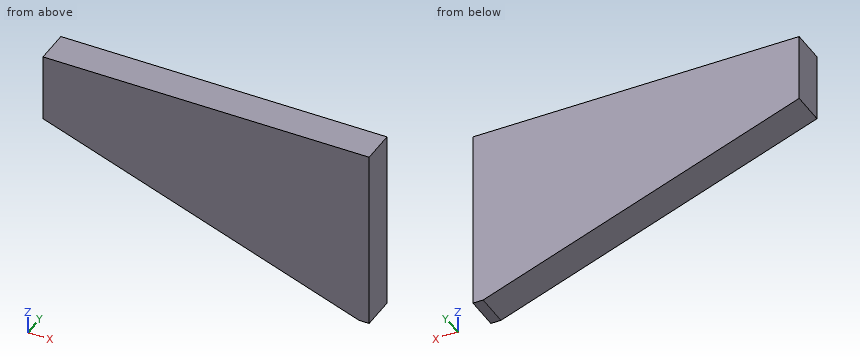
from build123d import *

# Parameters (mm, degrees)
BOX728_W               = 80
BOX728_H               = 6
BOX728_DEPTH           = 20
BOX728_PLACEMENT_ANGLE = 20
BOX724_W               = 57
BOX724_H               = 6
BOX724_DEPTH           = 32


with BuildPart() as krychle728:
    # Box728 → Box728 (new body)
    with BuildSketch(Plane.XY):
        with Locations((40, 3)):
            Rectangle(BOX728_W, BOX728_H)
    extrude(amount=BOX728_DEPTH)


with BuildPart() as krychle728_1:
    # Box728 placement: moved
    add(krychle728.part.moved(Location((-131.7, -24, 54.35))).rotate(Axis((-131.7, -24, 54.35), (0, 1, 0)), BOX728_PLACEMENT_ANGLE))


with BuildPart() as cut531:
    # Box724 → Box724 (new body)
    with BuildSketch(Plane(origin=(-122, -24, 52), x_dir=(1, 0, 0), z_dir=(0, 0, 1))):
        with Locations((28.5, 3)):
            Rectangle(BOX724_W, BOX724_H)
    extrude(amount=BOX724_DEPTH)

    # Cut531: cut Krychle728
    add(krychle728_1.part, mode=Mode.SUBTRACT)


solid = cut531.part
Geometry check sheet. Reference: the model listing, model coordinates, mm. Round coordinates to 2 decimals unless told otherwise and drop trailing zeros. Loops run counter-clockwise (first coordinate to the right, second up) from the corner with the lowest first, then second, coordinate; pieces in that order, holes last.
Item 1: Cross-section at A-A on y = -21.3. Record the boundary of the cut face in (x, z), then the cut area to 3 significant figures.
Item 2: Thickness scan on line 1 (Z direction, x = -68.5, y = -22.9); line 2 (Z direction, x = -75, y = -22.2). Record the ranges inside material, lowest first.
Item 3: Cross-section at B-B on z = 67. Record the boundary of the cut face in (x, y).
Item 4: Cross-section at C-C on x = -93. Record the boundary of the cut face in (y, z).
Answer sheet:
1. outline: (-122, 72.1) - (-66.77, 52) - (-65, 52) - (-65, 84) - (-122, 84) - close
1. area: 1,270 mm2
2. line 1: z = 52.63 to 84
2. line 2: z = 55 to 84
3. outline: (-107.98, -24) - (-65, -24) - (-65, -18) - (-107.98, -18) - close
4. outline: (-24, 61.55) - (-18, 61.55) - (-18, 84) - (-24, 84) - close
